Input: part model. Units: mm. Frame: model coordinates. A direction names the side the tool comes from. Round coordinates to 2 decimals unless told otherwise and drop trailing zeros. Order: outer loops, then holes, each group sorted by start corner. A loop starts at its lowest first (then second) coordinate and runs counter-clockwise, first axis right, second up. Notation, with made-up numbers: (64.25, 72) -> (70.25, 72) arc R22 ccw to (70.25, 79) -> close; hole circle Ø7 at (-12, -2.5). An arc over 180 degrees is marked (long way). Answer as CSV lines item,"result". Start each with the question number.
1) Access query for faces 1 (the face through (99, -6, 0)), 2 (the face through (140.48, -12.1, 5.92)), 3 (the face through (213.714, -23.407, 6.084)). Directions: +Z, -Z, +X, -X, +Y, -Y. A direction counts if a zero-diameter tool reaches every point of the face in a straight line with its end or side. Return the directions, or none.
2) Section query C-C, the plane z = 8.25. State how many separate pieces and enclosed holes the cut face has, and give its area (3 significant figures).
3) Section query B-B, the plane x = 42. Output: boundary loops of the cut face in (y, z), and give its area (3 significant figures).
4) First-contact query: P1, Ø4, axis at x = 122.5, z = 2.5, coming from the +Y side; P2, Ø6, axis at y = -0.5, z = 8.5, coming from the +X side; P3, Ø2, axis at y = 11.5, z = 2, coming from the +X side. Flat tips, straight axial feed; report the tip coordinate or a pass-through.
5) Section query A-A, the plane x = 93. Output: boundary loops of the cut face in (y, z), and give its area (3 significant figures).
6) Mould query, pull axis X, two halves, no side actions, for faces 4 (the face through (192.67, 22.35, 5.92)), 5 (the face through (140.69, 11.38, 5.92)), 6 (the face through (99, -6, 12)), 7 (the face through (30, 0, 6)). Classes: +X half, -X half, draft (parallel to the pull), parting line (faces both ways), or undercut.
7) Section query D-D, the plane x = 216. Output: boundary loops of the cut face in (y, z).
8) Line query: L1, parallel to Y at x = 186, z = 6.75; L2, parallel to Y at x = 166, z = 8.5; L3, parallel to Y at x = 0, z = 4.5. Output: solid intervals per line, ascending.
```python
from build123d import *

# Parameters (mm, degrees)
SKETCH_1_R           = 2.6
EXTRUDE_1_DEPTH      = 12
SKETCH_2_R           = 17
CUT_EXTRUDE_1_DEPTH  = 319.424245308
FILLET_1_R           = 50
SKETCH_7_R           = 21
CUT_EXTRUDE_6_DEPTH  = 319.424245308
SKETCH_15_R          = 48
CUT_EXTRUDE_12_DEPTH = 319.424245308
CUT_EXTRUDE_13_DEPTH = 234.372713636
CUT_EXTRUDE_14_DEPTH = 234.372713636
SKETCH_19_W          = 9.577046033
SKETCH_19_H          = 9.102233312
EXTRUDE_3_DEPTH      = 1
CUT_EXTRUDE_16_DEPTH = 234.372713636
FILLET_11_R          = 5
FILLET_12_R          = 15
FILLET_13_R          = 5


with BuildPart() as part:
    # 草图1 → 凸台-拉伸1 (new body)
    with BuildSketch(Plane.XY):
        with BuildLine():
            Line((0.975449173, 29.984137455), (231.02885683, 22.5))
            ThreePointArc((231.02885683, 22.5), (315, 0), (231.02885683, -22.5))
            Line((231.02885683, -22.5), (0.975449173, -29.984137455))
            ThreePointArc((0.975449173, -29.984137455), (-30, 0), (0.975449173, 29.984137455))
        make_face()
        with Locations((186, 18)):
            Circle(SKETCH_1_R, mode=Mode.SUBTRACT)
        with Locations(Location((186, -18, 0), (0, 0, 180))):
            Circle(SKETCH_1_R, mode=Mode.SUBTRACT)
        with Locations((216, -16.952376915)):
            Circle(SKETCH_1_R, mode=Mode.SUBTRACT)
    extrude(amount=EXTRUDE_1_DEPTH)

    # 草图2 → 切除-拉伸1 (cut, through all)
    with BuildSketch(Plane.XY.offset(12)):
        Circle(SKETCH_2_R)
    extrude(amount=-CUT_EXTRUDE_1_DEPTH, mode=Mode.SUBTRACT)

    # Fillet 1
    fillet_1_edges = [part.edges().sort_by_distance(p)[0] for p in [
        (231.02885683, 22.5, 6),
        (231.02885683, -22.5, 6),
    ]]
    fillet(fillet_1_edges, radius=FILLET_1_R)

    # 草图7 → 切除-拉伸6 (cut, through all)
    with BuildSketch(Plane.XY.offset(12)):
        with Locations((270, 0)):
            Circle(SKETCH_7_R)
    extrude(amount=-CUT_EXTRUDE_6_DEPTH, mode=Mode.SUBTRACT)

    # 草图15 → 切除-拉伸12 (cut, through all)
    with BuildSketch(Plane(origin=(0, 0, 0), x_dir=(-1, 0, 0), z_dir=(0, 0, -1))):
        with Locations((-270, 0)):
            Circle(SKETCH_15_R)
    extrude(amount=-CUT_EXTRUDE_12_DEPTH, mode=Mode.SUBTRACT)

    # 草图16 → 切除-拉伸13 (cut, through all)
    with BuildSketch(Plane(origin=(0, 0, 0), x_dir=(-1, 0, 0), z_dir=(0, 0, -1))):
        with BuildLine():
            ThreePointArc((-222, 0), (-224.338232659, 14.798750059), (-231.125125138, 28.155711755))
            ThreePointArc((-231.125125138, 28.155711755), (-223.636221951, 25.273493876), (-215.782692909, 23.62639569))
            ThreePointArc((-215.782692909, 23.62639569), (-220.419657795, 12.215374337), (-222, 0))
        make_face()
    extrude(amount=-CUT_EXTRUDE_13_DEPTH, mode=Mode.SUBTRACT)

    # 草图17 → 切除-拉伸14 (cut, through all)
    with BuildSketch(Plane(origin=(0, 0, 0), x_dir=(-1, 0, 0), z_dir=(0, 0, -1))):
        with BuildLine():
            ThreePointArc((-188.5, 2.750055906), (-191.110952969, 6.501128866), (-195.535274173, 5.355264285))
            Line((-195.535274173, 5.355264285), (-207.249830265, -8.293121713))
            ThreePointArc((-207.249830265, -8.293121713), (-207.697838632, -11.502932426), (-204.966217001, -13.247019458))
            Line((-204.966217001, -13.247019458), (-192.490456487, -13.217253727))
            ThreePointArc((-192.490456487, -13.217253727), (-189.668200744, -12.04231608), (-188.5, -9.217265111))
            Line((-188.5, -9.217265111), (-188.5, 2.750055906))
        make_face()
        with BuildLine():
            ThreePointArc((-178.455108958, 7.554652032), (-181.696939195, 8.110441149), (-183.5, 5.359561914))
            Line((-183.5, 5.359561914), (-183.5, -9.186248604))
            ThreePointArc((-183.5, -9.186248604), (-182.325050968, -12.018047861), (-179.490456487, -13.18623722))
            Line((-179.490456487, -13.18623722), (-163.845250629, -13.148909555))
            ThreePointArc((-163.845250629, -13.148909555), (-161.059570263, -11.244388724), (-161.807517222, -7.953827976))
            Line((-161.807517222, -7.953827976), (-178.455108958, 7.554652032))
        make_face()
        with BuildLine():
            Line((-155.98568473, 13.130157534), (-167.304455128, 13.15716282))
            ThreePointArc((-167.304455128, 13.15716282), (-170.101829155, 11.259302243), (-169.356503805, 7.96208124))
            Line((-169.356503805, 7.96208124), (-156.726521389, -3.803694429))
            ThreePointArc((-156.726521389, -3.803694429), (-152.404081073, -4.544746584), (-150, -0.876907605))
            Line((-150, -0.876907605), (-150, 7.130174611))
            ThreePointArc((-150, 7.130174611), (-151.752301116, 11.367751063), (-155.98568473, 13.130157534))
        make_face()
        with BuildLine():
            ThreePointArc((-136.48568473, 13.083632773), (-140.737576452, 11.331348735), (-142.5, 7.083649851))
            Line((-142.5, 7.083649851), (-142.5, -8.086038582))
            ThreePointArc((-142.5, -8.086038582), (-140.427707672, -12.139250616), (-135.928588884, -12.832686568))
            Line((-135.928588884, -12.832686568), (-81.584472606, 5.158314378))
            ThreePointArc((-81.584472606, 5.158314378), (-78.891840256, 9.587602802), (-82.832057986, 12.955621382))
            Line((-82.832057986, 12.955621382), (-136.48568473, 13.083632773))
        make_face()
        with BuildLine():
            ThreePointArc((-97.462029586, -7.12436313), (-99.534348383, -10.443548142), (-96.561920261, -12.988379256))
            Line((-96.561920261, -12.988379256), (-32.822141486, -12.836303465))
            ThreePointArc((-32.822141486, -12.836303465), (-29.654019481, -11.265809006), (-28.969133823, -7.796748397))
            ThreePointArc((-28.969133823, -7.796748397), (-30, 0), (-28.969133823, 7.796748397))
            ThreePointArc((-28.969133823, 7.796748397), (-30.059408875, 11.719799736), (-34.022287252, 12.655014403))
            Line((-34.022287252, 12.655014403), (-97.462029586, -7.12436313))
        make_face()
    extrude(amount=-CUT_EXTRUDE_14_DEPTH, mode=Mode.SUBTRACT)

    # 草图21 → 切除-拉伸16 (cut, through all)
    with BuildSketch(Plane.XY.offset(12)):
        with BuildLine():
            Line((225.346998742, -17.609925571), (193.471450892, 23.72182406))
            Line((193.471450892, 23.72182406), (207.853731728, 23.253937199))
            ThreePointArc((207.853731728, 23.253937199), (211.825615161, 23.282573441), (215.782692909, 23.62639569))
            ThreePointArc((215.782692909, 23.62639569), (220.419657795, 12.215374337), (222, 0))
            ThreePointArc((222, 0), (222.844172892, -8.962587227), (225.346998742, -17.609925571))
        make_face()
    extrude(amount=-CUT_EXTRUDE_16_DEPTH, mode=Mode.SUBTRACT)

    # 圆角11
    # the kernel refuses this fillet: 5 mm, written as the material it takes off along each edge
    with BuildSketch(Plane(origin=(231.125125138, -28.155711755, -30.280019258), x_dir=(-0.9472337070589926, 0.3205437633323705, 0), z_dir=(0, 0, 1))) as fillet_11_piece_1:
        with BuildLine():
            CenterArc((12.717608088, -4.963189315), FILLET_11_R, 96.956749804, 123.184808142)
            ThreePointArc((8.895338078, -8.186580691), (4.706429893, -3.812127139), (0, 0))
            ThreePointArc((0, 0), (6.056003852, -0.368106853), (12.112007703, 0))
        make_face()
    extrude(amount=72.560038515, mode=Mode.SUBTRACT)

    # 圆角12
    fillet_12_edges = [part.edges().sort_by_distance(p)[0] for p in [
        (193.471450892, 23.72182406, 6),
    ]]
    fillet(fillet_12_edges, radius=FILLET_12_R)

    # 圆角13
    fillet_13_edges = [part.edges().sort_by_distance(p)[0] for p in [
        (225.346030547, -17.608670152, 6),
    ]]
    fillet(fillet_13_edges, radius=FILLET_13_R)


with BuildPart() as body_2:
    # 草图19 → 凸台-拉伸3 (new body)
    with BuildSketch(Plane(origin=(0, 0, 0), x_dir=(0, 0, -1), z_dir=(1, 0, 0))):
        with Locations((4.788523017, -4.551116656)):
            Rectangle(SKETCH_19_W, SKETCH_19_H)
    extrude(amount=EXTRUDE_3_DEPTH)


solid = part.part
```
Findings:
1,face 1,"-Z, +X, -X, +Y, -Y"
1,face 2,"+Z, -Z"
1,face 3,"+Z, -Z, -Y"
2,separate pieces,"1"
2,enclosed holes,"9"
2,area,"8,630 mm^2"
3,outline,"(-28.65, 0) -> (-12.86, 0) -> (-12.86, 12) -> (-28.65, 12) -> close; (10.17, 0) -> (28.65, 0) -> (28.65, 12) -> (10.17, 12) -> close"
3,area,"411 mm^2"
4,P1,"stops at y = 26.1"
4,P2,"stops at x = 214.47"
4,P3,"stops at x = 203.67"
5,outline,"(-26.99, 0) -> (-12.98, 0) -> (-12.98, 12) -> (-26.99, 12) -> close; (-5.73, 0) -> (1.38, 0) -> (1.38, 12) -> (-5.73, 12) -> close; (12.98, 0) -> (26.99, 0) -> (26.99, 12) -> (12.98, 12) -> close"
5,area,"422 mm^2"
6,face 4,"+X half"
6,face 5,"undercut"
6,face 6,"draft"
6,face 7,"undercut"
7,outline,"(-23.65, 0) -> (-19.55, 0) -> (-19.55, 12) -> (-23.65, 12) -> close; (-14.35, 0) -> (-5.49, 0) -> (-5.49, 12) -> (-14.35, 12) -> close"
8,L1,"y = -23.96 to -20.6, -15.4 to 15.4, 20.6 to 23.96"
8,L2,"y = -24.62 to -13.15, -4.05 to 4.84, 13.15 to 24.62"
8,L3,"y = -30 to -17, 17 to 30"
